from build123d import *

# Parameters (mm, degrees)
BOSS_EXTRUDE1_DEPTH = 5
SKETCH3_R           = 2.5
CUT_EXTRUDE1_DEPTH  = 10
FILLET7_R           = 3


with BuildPart() as part:
    # Sketch1 → Revolve1 (revolve)
    with BuildSketch(Plane(origin=(0, 0, 0), x_dir=(1, 0, 0), z_dir=(0, 1, 0))):
        with BuildLine():
            Line((-32.5, 0), (32.5, 0))
            ThreePointArc((32.5, 0), (0, -32.5), (-32.5, 0))
        make_face()
    revolve(axis=Axis((-32.5, 0, 0), (1, 0, 0)))

    # Sketch2 → Boss-Extrude1 (add, symmetric)
    with BuildSketch(Plane.XY):
        with BuildLine():
            Line((-4.287633392, 40), (-4.287633392, 25))
            Line((-4.287633392, 25), (5.712366608, 25))
            Line((5.712366608, 25), (5.712366608, 40))
            ThreePointArc((5.712366608, 40), (0.712366608, 45), (-4.287633392, 40))
        make_face()
    extrude(amount=BOSS_EXTRUDE1_DEPTH, both=True)

    # Sketch3 → Cut-Extrude1 (cut)
    with BuildSketch(Plane.XY.offset(5)):
        with Locations((0.712366608, 40)):
            Circle(SKETCH3_R)
    extrude(amount=-CUT_EXTRUDE1_DEPTH, mode=Mode.SUBTRACT)

    # Fillet7
    fillet7_edges = [part.edges().sort_by_distance(p)[0] for p in [
        (-4.287633392, 32.21593084, 0),
        (5.712366608, 31.994044254, 0),
        (-4.287633392, 35.912779455, -5),
        (5.712366608, 35.800465719, -5),
        (-4.287633392, 35.912779455, 5),
        (5.712366608, 35.800465719, 5),
        (0.72116611, 32.104982782, -5),
        (0.72116611, 32.104982782, 5),
    ]]
    fillet(fillet7_edges, radius=FILLET7_R)


solid = part.part
Work out the finished part from the listing and answer in its coordinate system (mm). Round coordinates to 2 decimals unless told otherwise and drop trailing zeros. Write each loop counter-clockwise with the first axis right and the second up, starting at its lowest first coordinate (ties: lowest second). Pieces come first, ordered by that corner, then holes. Notation, with made-up numbers: (73.25, -16.75) -> (89.25, -16.75) arc R12 ccw to (89.25, -0.75) -> close; hole circle Ø10 at (39, 8.25). An arc over 180 degrees is marked (long way). Answer as CSV lines item,"result". Start each with the question number.
(1) Find the intervals of material crossed by probe 1 along X at (y, z) = (40, 0.5); probe 2 along Y at (x, z) = (1, 3); probe 3 along X at (y, z) = (-4.5, -10.5), in increasing order.
(2) Each of these flat-tipped pins is pushed along its axis until it touches: pin 1 (4.5 mm diameter, centred on x = 0.5, y = 36.5, fed in from -Z); pin 2 (1 mm diameter, centred on y = -14, z = -5.5, fed in from -X); pin 3 (6 mm diameter, centred on x = 21.5, z = 6.5, fed in from +Y). Where does it stop, or does it pass through?
(3) The mould has two halves that part along Y. Classify faces 1 (the cylindrical face through (0.8, 45, 0)), 2 (the cylindrical face through (0.17, 37.56, 0.07)): +Y half, -Y half, draft (parallel to the pull), parting line (faces both ways), or undercut.
(4) The part is cut by section B-B, the plane y = -20. Give the vertices of the cut face in (x, z), then the cut area to 3 significant figures.
(5) The part is cut by section A-A, the plane z = -15. Give the vertices of the cut face in (x, y), then the cut area to 3 significant figures.
Output values:
1,probe 1,"x = -4.29 to -1.79, 3.21 to 5.71"
1,probe 2,"y = -32.35 to 37.52, 42.48 to 44.83"
1,probe 3,"x = -30.43 to 30.43"
2,pin 1,"stops at z = -5.02"
2,pin 2,"stops at x = -29.07"
2,pin 3,"stops at y = 26.03"
3,face 1,"+Y half"
3,face 2,"undercut"
4,outline,"circle Ø51.23 at (0, 0)"
4,area,"2,060 mm²"
5,outline,"circle Ø57.66 at (0, 0)"
5,area,"2,610 mm²"
